Check sheet for the modelled part. Datum: model origin and axes. Units: mm. Round coordinates to 2 decimals unless told otherwise and drop trailing zeros. Order: outer loops, then holes, each group sorted by start corner. A loop starts at its lowest first (then second) coordinate and runs counter-clockwise, first axis right, second up.
Q1. Cross-section at C-C on y = -186. Record the cut outline in (x, z) (3 decimals).
Q2. Cross-section at A-A on z = 0.85. Record the cut outline in (x, y).
Q3. Mould release check, pull along X, two halves, no side actions. Record for faces 1 (the cylindrical face through (2.502, -215.886, 1.565)), 2 (the cylindrical face through (-5.83, -241.23, 1.57)), 3 (the flat face through (-2, -218, 0)): +X half, -X half, draft (parallel to the pull), parting line (faces both ways), or undercut.
Q4. Scan lines: probe 1 along X at (y, z) = (-182, 1.9); probe 2 along Y at (x, z) = (0, 2.3); probe 3 along Y at (x, z) = (139.7, 1.45). Record each from-to range of solid material in increasing order.
Q5. Depth check by flat-ended pin: P1, Ø1.5, axis at x = 166, z = 2.5, coming from the +Y side. Enter the tip coordinate at first touch or a pass-through.
Q6. Cross-section at D-D on x = -57.5. Record the cut outline in (y, z) (3 decimals), then the cut area to 3 significant figures.
Q7. Cross-section at B-B on y = -146.5. Record the cut outline in (x, z) (3 decimals), then the cut area to 3 significant figures.
from build123d import *

# Parameters (mm, degrees)
SKETCH1_R           = 2.0193
SKETCH1_R_2         = 3.2639
BOSS_EXTRUDE1_DEPTH = 3.175
FILLET1_R           = 2.54


with BuildPart() as part:
    # Sketch1 → Boss-Extrude1 (new body)
    with BuildSketch(Plane.XY):
        with BuildLine():
            Line((-190.5, -101.6), (-218.867836833, -101.6))
            ThreePointArc((-218.867836833, -101.6), (0, -241.3), (218.867836833, -101.6))
            Line((218.867836833, -101.6), (190.5, -101.6))
            ThreePointArc((190.5, -101.6), (0, -215.9), (-190.5, -101.6))
        make_face()
        with Locations((-139.7, -177.8)):
            Circle(SKETCH1_R, mode=Mode.SUBTRACT)
        with Locations((-197.973407305, -114.3)):
            Circle(SKETCH1_R_2, mode=Mode.SUBTRACT)
        with Locations((0, -228.6)):
            Circle(SKETCH1_R_2, mode=Mode.SUBTRACT)
        with Locations((139.7, -177.8)):
            Circle(SKETCH1_R, mode=Mode.SUBTRACT)
        with Locations((197.973407305, -114.3)):
            Circle(SKETCH1_R_2, mode=Mode.SUBTRACT)
    extrude(amount=BOSS_EXTRUDE1_DEPTH)

    # Fillet1
    fillet1_edges = [part.edges().sort_by_distance(p)[0] for p in [
        (190.5, -101.6, 1.5875),
        (218.867836833, -101.6, 1.5875),
    ]]
    fillet(fillet1_edges, radius=FILLET1_R)


solid = part.part
Results found:
1. outline: (-153.72, 0) - (-109.621, 0) - (-109.621, 3.175) - (-153.72, 3.175) - close; (109.621, 0) - (153.72, 0) - (153.72, 3.175) - (109.621, 3.175) - close
2. outline: (-218.87, -101.6) arc R241.3 ccw to (217.14, -105.25) arc R2.54 ccw to (214.85, -101.6) - (192.02, -101.6) arc R2.54 ccw to (189.79, -102.93) arc R215.9 cw to (-190.5, -101.6) - close; hole circle Ø6.53 at (-197.97, -114.3); hole circle Ø4.04 at (-139.7, -177.8); hole circle Ø6.53 at (0, -228.6); hole circle Ø4.04 at (139.7, -177.8); hole circle Ø6.53 at (197.97, -114.3)
3. face 1: undercut
3. face 2: parting line
3. face 3: draft
4. probe 1: x = -158.44 to -116.14, 116.14 to 158.44
4. probe 2: y = -241.3 to -231.86, -225.34 to -215.9
4. probe 3: y = -196.75 to -179.82, -175.78 to -164.61
5. P1: stops at y = -137.14
6. outline: (-234.349, 0) - (-208.102, 0) - (-208.102, 3.175) - (-234.349, 3.175) - close
6. area: 83.3 mm2
7. outline: (-191.738, 0) - (-158.589, 0) - (-158.589, 3.175) - (-191.738, 3.175) - close; (158.589, 0) - (191.738, 0) - (191.738, 3.175) - (158.589, 3.175) - close
7. area: 210 mm2
